Can you work these out from the model? Positions are in its coordinate system, mm. A direction names the side the tool comes from. Give positions to 0.01 mm unless a question says otherwise; leave off trailing zeros. Write each loop counter-clockwise with the first axis right and the second up, starting at its lowest first coordinate (ties: lowest second). Pieces come first, ordered by that corner, then holes. Notation, with made-up numbers: (83.5, 40) - (120.5, 40) arc R20 cw to (120.5, 71) - close; hole circle Ø3 at (82, -3). An arc over 180 degrees is marked (long way). Use a Markdown table: item, result. Add a question column.
```python
from build123d import *

# Parameters (mm, degrees)
BASE_FLANGE1_DEPTH           = 574.9
EDGE_FLANGE1_DEPTH           = 767
F_7_0_7_DIAMETER_HOLE1_D     = 7
F_7_0_7_DIAMETER_HOLE1_DEPTH = 2
LPATTERN1_COUNT              = 7
LPATTERN1_PITCH              = 90.816666667
MIRROR1_COPY_1_D             = 7
MIRROR1_COPY_1_DEPTH         = 2
MIRROR1_COPY_2_D             = 7
MIRROR1_COPY_2_DEPTH         = 2
MIRROR1_COPY_3_D             = 7
MIRROR1_COPY_3_DEPTH         = 2
MIRROR1_COPY_4_D             = 7
MIRROR1_COPY_4_DEPTH         = 2
MIRROR1_COPY_5_D             = 7
MIRROR1_COPY_5_DEPTH         = 2
MIRROR1_COPY_6_D             = 7
MIRROR1_COPY_6_DEPTH         = 2
F_7_0_7_DIAMETER_HOLE2_D     = 7
LPATTERN2_COUNT              = 7
LPATTERN2_PITCH              = 121.166666667
M8_CLEARANCE_HOLE1_D         = 9
LPATTERN3_COUNT              = 6
LPATTERN3_PITCH              = 129
F_7_0_7_DIAMETER_HOLE3_D     = 7
SKETCH21_R                   = 26
CUT_EXTRUDE1_DEPTH           = 20
M6_CLEARANCE_HOLE1_D         = 6.6
M5_CLEARANCE_HOLE1_D         = 5.8
SKETCH26_R                   = 10.75
CUT_EXTRUDE2_DEPTH           = 10
M16_CLEARANCE_HOLE1_D        = 17
CUT_EXTRUDE3_DEPTH           = 10
M5_CLEARANCE_HOLE2_D         = 5.8
FILLET1_R                    = 3


# Sheet-metal steps are written as plain solids
with BuildPart() as part:
    # Sketch1 → Base-Flange1 (new body)
    with BuildSketch(Plane(origin=(0, 0, 0), x_dir=(1, 0, 0), z_dir=(0, 1, 0))):
        with BuildLine():
            Line((25, 387.5), (4, 387.5))
            ThreePointArc((4, 387.5), (1.171572875, 386.328427125), (0, 383.5))
            Line((0, 383.5), (0, -383.5))
            ThreePointArc((0, -383.5), (1.171572875, -386.328427125), (4, -387.5))
            Line((4, -387.5), (25, -387.5))
            Line((25, -387.5), (25, -385.5))
            Line((25, -385.5), (4, -385.5))
            ThreePointArc((4, -385.5), (2.585786438, -384.914213562), (2, -383.5))
            Line((2, -383.5), (2, 383.5))
            ThreePointArc((2, 383.5), (2.585786438, 384.914213562), (4, 385.5))
            Line((4, 385.5), (25, 385.5))
            Line((25, 385.5), (25, 387.5))
        make_face()
    extrude(amount=BASE_FLANGE1_DEPTH)

    # Edge-Flange1 section (across the edge) → Edge-Flange1 (add)
    with BuildSketch(Plane(origin=(2, 576.9, -383.5), x_dir=(0, -1, 0), z_dir=(0, 0, 1))):
        with BuildLine():
            Line((-2, 2), (-2, 23))
            Line((-2, 23), (0, 23))
            Line((0, 23), (0, 2))
            ThreePointArc((0, 2), (0.585786438, 0.585786438), (2, 0))
            Line((2, 0), (2, -2))
            ThreePointArc((2, -2), (-0.828427125, -0.828427125), (-2, 2))
        make_face()
    extrude(amount=EDGE_FLANGE1_DEPTH)

    # Ø7.0 (7) Diameter Hole1
    with Locations(Plane(origin=(0, 0, 385.5), x_dir=(-1, 0, 0), z_dir=(0, 0, -1))):
        with Locations((-16.5, 559.9)):
            f_7_0_7_diameter_hole1 = Hole(F_7_0_7_DIAMETER_HOLE1_D / 2, depth=F_7_0_7_DIAMETER_HOLE1_DEPTH)

    # LPattern1: Ø7.0 (7) Diameter Hole1 ×7
    with Locations(*[(0, -i * LPATTERN1_PITCH, 0) for i in range(1, LPATTERN1_COUNT)]):
        add(f_7_0_7_diameter_hole1, mode=Mode.SUBTRACT)

    # Mirror1: Ø7.0 (7) Diameter Hole1 across plane
    add(f_7_0_7_diameter_hole1.mirror(Plane.XY), mode=Mode.SUBTRACT)

    # Mirror1 copy 1
    with Locations(Plane(origin=(0, -90.816666667, -385.5), x_dir=(-1, 0, 0), z_dir=(0, 0, 1))):
        with Locations((-16.5, -559.9)):
            Hole(MIRROR1_COPY_1_D / 2, depth=MIRROR1_COPY_1_DEPTH)

    # Mirror1 copy 2
    with Locations(Plane(origin=(0, -181.633333333, -385.5), x_dir=(-1, 0, 0), z_dir=(0, 0, 1))):
        with Locations((-16.5, -559.9)):
            Hole(MIRROR1_COPY_2_D / 2, depth=MIRROR1_COPY_2_DEPTH)

    # Mirror1 copy 3
    with Locations(Plane(origin=(0, -272.45, -385.5), x_dir=(-1, 0, 0), z_dir=(0, 0, 1))):
        with Locations((-16.5, -559.9)):
            Hole(MIRROR1_COPY_3_D / 2, depth=MIRROR1_COPY_3_DEPTH)

    # Mirror1 copy 4
    with Locations(Plane(origin=(0, -363.266666667, -385.5), x_dir=(-1, 0, 0), z_dir=(0, 0, 1))):
        with Locations((-16.5, -559.9)):
            Hole(MIRROR1_COPY_4_D / 2, depth=MIRROR1_COPY_4_DEPTH)

    # Mirror1 copy 5
    with Locations(Plane(origin=(0, -454.083333333, -385.5), x_dir=(-1, 0, 0), z_dir=(0, 0, 1))):
        with Locations((-16.5, -559.9)):
            Hole(MIRROR1_COPY_5_D / 2, depth=MIRROR1_COPY_5_DEPTH)

    # Mirror1 copy 6
    with Locations(Plane(origin=(0, -544.9, -385.5), x_dir=(-1, 0, 0), z_dir=(0, 0, 1))):
        with Locations((-16.5, -559.9)):
            Hole(MIRROR1_COPY_6_D / 2, depth=MIRROR1_COPY_6_DEPTH)

    # Ø7.0 (7) Diameter Hole2 (through all)
    with Locations(Plane(origin=(0, 578.9, 0), x_dir=(1, 0, 0), z_dir=(0, 1, 0))):
        with Locations((16.5, -363.5)):
            f_7_0_7_diameter_hole2 = Hole(F_7_0_7_DIAMETER_HOLE2_D / 2)

    # LPattern2: Ø7.0 (7) Diameter Hole2 ×7
    with Locations(*[(0, 0, -i * LPATTERN2_PITCH) for i in range(1, LPATTERN2_COUNT)]):
        add(f_7_0_7_diameter_hole2, mode=Mode.SUBTRACT)

    # M8 Clearance Hole1 (through all)
    with Locations(Plane(origin=(2, 0, 0), x_dir=(0, 0, -1), z_dir=(1, 0, 0))):
        with Locations((-322.5, 15)):
            m8_clearance_hole1 = Hole(M8_CLEARANCE_HOLE1_D / 2)

    # LPattern3: M8 Clearance Hole1 ×6
    with Locations(*[(0, 0, -i * LPATTERN3_PITCH) for i in range(1, LPATTERN3_COUNT)]):
        add(m8_clearance_hole1, mode=Mode.SUBTRACT)

    # Ø7.0 (7) Diameter Hole3 (through all)
    with Locations(Plane(origin=(0, 578.9, 0), x_dir=(1, 0, 0), z_dir=(0, 1, 0))):
        with Locations((16.5, 280), (16.5, 225)):
            Hole(F_7_0_7_DIAMETER_HOLE3_D / 2)

    # Sketch21 → Cut-Extrude1 (cut)
    with BuildSketch(Plane(origin=(2, 0, 0), x_dir=(0, 0, -1), z_dir=(1, 0, 0))):
        with Locations((0, 506.9)):
            Circle(SKETCH21_R)
    extrude(amount=-CUT_EXTRUDE1_DEPTH, mode=Mode.SUBTRACT)

    # M6 Clearance Hole1 (through all)
    with Locations(Plane(origin=(2, 0, 0), x_dir=(0, 0, -1), z_dir=(1, 0, 0))):
        with Locations((-33.875, 506.9), (-16.9375, 536.236610553), (-16.9375, 477.563389447), (16.9375, 477.563389447), (16.9375, 536.236610553), (33.875, 506.9)):
            Hole(M6_CLEARANCE_HOLE1_D / 2)

    # M5 Clearance Hole1 (through all)
    with Locations(Plane.ZY):
        with Locations((-69.646446609, 453.961547076), (-92, 476.290170104), (-92, 536.731392746), (0, 453.961547076), (69.646446609, 453.961547076), (92, 476.290170104), (92, 536.731392746), (69.646446609, 559.060015773), (0, 559.060015773), (-69.646446609, 559.060015773)):
            Hole(M5_CLEARANCE_HOLE1_D / 2)

    # Sketch26 → Cut-Extrude2 (cut)
    with BuildSketch(Plane(origin=(2, 0, 0), x_dir=(0, 0, -1), z_dir=(1, 0, 0))):
        with Locations((68, 506.9)):
            Circle(SKETCH26_R)
    extrude(amount=-CUT_EXTRUDE2_DEPTH, mode=Mode.SUBTRACT)

    # M16 Clearance Hole1 (through all)
    with Locations(Plane(origin=(2, 0, 0), x_dir=(0, 0, -1), z_dir=(1, 0, 0))):
        with Locations((-70, 506.9)):
            Hole(M16_CLEARANCE_HOLE1_D / 2)

    # Sketch29 → Cut-Extrude3 (cut)
    with BuildSketch(Plane(origin=(2, 0, 0), x_dir=(0, 0, -1), z_dir=(1, 0, 0))):
        with BuildLine():
            Line((183.5, 80), (328.5, 80))
            ThreePointArc((328.5, 80), (332.035533906, 81.464466094), (333.5, 85))
            Line((333.5, 85), (333.5, 128))
            ThreePointArc((333.5, 128), (332.035533906, 131.535533906), (328.5, 133))
            Line((328.5, 133), (183.5, 133))
            ThreePointArc((183.5, 133), (179.964466094, 131.535533906), (178.5, 128))
            Line((178.5, 128), (178.5, 85))
            ThreePointArc((178.5, 85), (179.964466094, 81.464466094), (183.5, 80))
        make_face()
    extrude(amount=-CUT_EXTRUDE3_DEPTH, mode=Mode.SUBTRACT)

    # M5 Clearance Hole2 (through all)
    with Locations(Plane(origin=(2, 0, 0), x_dir=(0, 0, -1), z_dir=(1, 0, 0))):
        with Locations((256, 138.999355653), (173.5, 138.999355653), (338.5, 138.999355653), (338.5, 74.000644347), (259.364988053, 74.000644347), (173.5, 74.000644347)):
            Hole(M5_CLEARANCE_HOLE2_D / 2)

    # Fillet1
    fillet1_edges = [part.edges().sort_by_distance(p)[0] for p in [
        (25, 0, -386.5),
        (25, 0, 386.5),
        (25, 574.9, -386.5),
        (25, 577.9, -383.5),
        (25, 577.9, 383.5),
        (25, 574.9, 386.5),
    ]]
    fillet(fillet1_edges, radius=FILLET1_R)


solid = part.part
```
Q1. I'm going to push flat-ended pins straight in: P1, Ø3, axis at y = 105, z = 280.5, coming from the +X side; P2, Ø3, axis at x = 17.5, z = 74, coming from the -Y side; P3, Ø2, axis at x = 14, y = 577, coming from the +Z side. Where does each tip first touch, or does it pass through?
Q2. Suppose I cut it at B-B (x = 8.75). Please give me the cut outline in (y, z), and give its area (3 significant figures).
Q3. Suppose I cut it at C-C (z = -47.5). Please give me the cut outline in (x, y).
Q4. Suppose I cut it at D-D (y = 352.5). Please give me the cut outline in (x, z), and give its area (3 significant figures).
Q5. If we mould it in two halves opening along Z, with no side actions, what happens to faces 4 (the flat face through (15, 576.9, -5)), 5 (the cylindrical face through (1.01, 517.56, -66.6)), 6 (the flat face through (15, 283, -387.5)), 7 (the flat face through (15, 283, 385.5))? For each: released by +Z, released by -Z, zero draft, split by the parting line, or undercut.
Q6. Suppose I cut it at A-A (y = 94.5). Please give me the cut outline in (x, z).
Q7. If I drill on probe 1 along Y at (x, z) = (0.55, -92); probe 2 along Z at (x, y) = (19, 27); probe 3 along X at (y, z) = (39, 126), over which ranges is the centre line in solid material (lowest first)? Write a range as [from, to].
Q8. On a 3-axis mill with a long thin cutter (end or side, diameter ignored), from which of +Z, -Z, +X, -X, +Y, -Y can I reach the whole of each face in a straight line? I mean faces 1 (the flat face through (14, 283, -385.5)), 2 (the flat face through (2, 283, 5)), 3 (the cylindrical face through (1.01, 481.52, 5.64)). Say none if no direction works.
Derived:
| question | item | result |
|---|---|---|
| 1 | P1 | x = 2 |
| 1 | P2 | y = 576.9 |
| 1 | P3 | z = 383.5 |
| 2 | outline | (0, -387.5) - (574.9, -387.5) - (574.9, -385.5) - (0, -385.5) - close; (0, 385.5) - (574.9, 385.5) - (574.9, 387.5) - (0, 387.5) - close; (576.9, -383.5) - (578.9, -383.5) - (578.9, 383.5) - (576.9, 383.5) - close |
| 2 | area | 3,830 mm² |
| 3 | outline | (0, 0) - (2, 0) - (2, 574.9) arc R2 cw to (4, 576.9) - (25, 576.9) - (25, 578.9) - (4, 578.9) arc R4 ccw to (0, 574.9) - close |
| 4 | outline | (0, -383.5) arc R4 ccw to (4, -387.5) - (25, -387.5) - (25, -385.5) - (4, -385.5) arc R2 cw to (2, -383.5) - (2, 383.5) arc R2 cw to (4, 385.5) - (25, 385.5) - (25, 387.5) - (4, 387.5) arc R4 ccw to (0, 383.5) - close |
| 4 | area | 1,640 mm² |
| 5 | face 4 | zero draft |
| 5 | face 5 | undercut |
| 5 | face 6 | released by -Z |
| 5 | face 7 | undercut |
| 6 | outline | (0, -383.5) arc R4 ccw to (4, -387.5) - (25, -387.5) - (25, -385.5) - (4, -385.5) arc R2 cw to (2, -383.5) - (2, -333.5) - (0, -333.5) - close; (0, -178.5) - (2, -178.5) - (2, 383.5) arc R2 cw to (4, 385.5) - (25, 385.5) - (25, 387.5) - (4, 387.5) arc R4 ccw to (0, 383.5) - close |
| 7 | probe 1 | [0, 473.39], [479.19, 533.83], [539.63, 576.92] |
| 7 | probe 2 | [-387.5, -385.5], [385.5, 387.5] |
| 7 | probe 3 | [0, 2] |
| 8 | face 1 | +X, +Y, -Y |
| 8 | face 2 | +X, -Y |
| 8 | face 3 | +X, -X |
